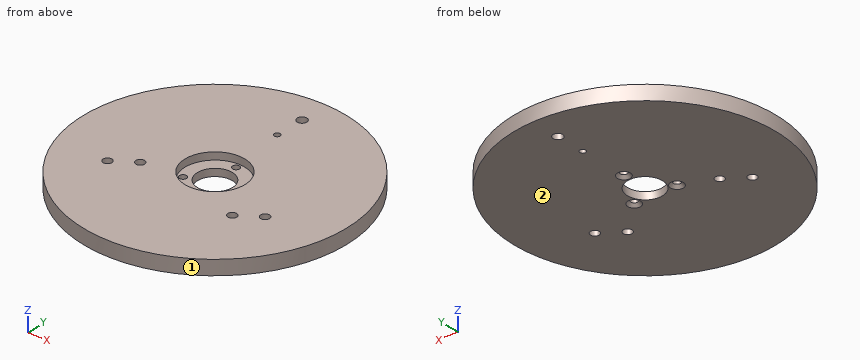
from build123d import *

# Parameters (mm, degrees)
SKETCH1_R                                       = 45
BOSS_EXTRUDE1_DEPTH                             = 5
F_20_5_20_5_DIAMETER_HOLE1_D                    = 20.5
F_20_5_20_5_DIAMETER_HOLE1_DEPTH                = 2.5
F_12_0_12_DIAMETER_HOLE1_D                      = 12
CSK_FOR_M2_FLAT_HEAD_MACHINE_SCREW1_D           = 2.4
CSK_FOR_M2_FLAT_HEAD_MACHINE_SCREW1_DEPTH       = 22.75
CSK_FOR_M2_FLAT_HEAD_MACHINE_SCREW1_CSINK_D     = 4.4
CSK_FOR_M2_FLAT_HEAD_MACHINE_SCREW1_CSINK_ANGLE = 90
CSK_FOR_M2_FLAT_HEAD_MACHINE_SCREW1_TIP         = 0.721032743
M4X0_7_TAPPED_HOLE1_D                           = 3.3
SKETCH15_R                                      = 1.5
M3_TAPPED_HOLE_DEPTH                            = 124.895116934
SKETCH16_R                                      = 1
F_2MM_PIN_DEPTH                                 = 124.895116934


with BuildPart() as part:
    # Sketch1 → Boss-Extrude1 (new body)
    with BuildSketch(Plane.XY.offset(39.5)):
        with Locations((-40, 45)):
            Circle(SKETCH1_R)
    extrude(amount=-BOSS_EXTRUDE1_DEPTH)

    # Ø20.5 (20.5) Diameter Hole1
    with Locations(Plane.XY.offset(39.5)):
        with Locations((-40, 45)):
            Hole(F_20_5_20_5_DIAMETER_HOLE1_D / 2, depth=F_20_5_20_5_DIAMETER_HOLE1_DEPTH)

    # Ø12.0 (12) Diameter Hole1 (through all)
    with Locations(Plane.XY.offset(39.5)):
        with Locations((-40, 45)):
            Hole(F_12_0_12_DIAMETER_HOLE1_D / 2)

    # CSK for M2 Flat Head Machine Screw1
    with Locations(Plane(origin=(0, 0, 34.5), x_dir=(1, 0, 0), z_dir=(0, 0, -1))):
        with Locations((-40, -53.5), (-32.638784068, -40.75), (-47.361215932, -40.75)):
            CounterSinkHole(CSK_FOR_M2_FLAT_HEAD_MACHINE_SCREW1_D / 2, CSK_FOR_M2_FLAT_HEAD_MACHINE_SCREW1_CSINK_D / 2, depth=CSK_FOR_M2_FLAT_HEAD_MACHINE_SCREW1_DEPTH, counter_sink_angle=CSK_FOR_M2_FLAT_HEAD_MACHINE_SCREW1_CSINK_ANGLE)
            with Locations((0, 0, -(CSK_FOR_M2_FLAT_HEAD_MACHINE_SCREW1_DEPTH + CSK_FOR_M2_FLAT_HEAD_MACHINE_SCREW1_TIP / 2))):  # 118° drill point
                Cone(0, CSK_FOR_M2_FLAT_HEAD_MACHINE_SCREW1_D / 2, CSK_FOR_M2_FLAT_HEAD_MACHINE_SCREW1_TIP, mode=Mode.SUBTRACT)

    # M4x0.7 Tapped Hole1 (through all)
    with Locations(Plane.XY.offset(39.5)):
        with Locations((-40, 80)):
            Hole(M4X0_7_TAPPED_HOLE1_D / 2)

    # Sketch15 → M3 Tapped Hole (cut, through all)
    with BuildSketch(Plane.XY.offset(39.5)):
        with Locations((-58, 36)):
            Circle(SKETCH15_R)
        with Locations((-65, 31)):
            Circle(SKETCH15_R)
        with Locations((-15, 36)):
            Circle(SKETCH15_R)
        with Locations((-22, 31)):
            Circle(SKETCH15_R)
    extrude(amount=-M3_TAPPED_HOLE_DEPTH, mode=Mode.SUBTRACT)

    # Sketch16 → 2mm Pin (cut, through all)
    with BuildSketch(Plane.XY.offset(39.5)):
        with Locations((-40, 70)):
            Circle(SKETCH16_R)
    extrude(amount=-F_2MM_PIN_DEPTH, mode=Mode.SUBTRACT)


solid = part.part
Geometry: final body of the model. Coordinates: model frame, mm. Face numbers are marked on the shaded views. Give positions to 0.01 mm unless a question says otherwise; leave off trailing zeros. Loops run counter-clockwise (first coordinate to the right, second up) from the corner with the lowest first, then second, coordinate; pieces in that order, holes last. Notation, with made-up numbers: (74, 65) - (109, 65) arc R14 cw to (109, 78) - close; hole circle Ø6 at (76.5, 78). An arc over 180 degrees is marked (long way). One line per question, with ' | ' between items. Start each with the question number.
(1) Pull-direction query (Y, two-part tool) for the marked faces 1 and 2; classes: released by +Y, released by -Y, zero draft, split by the parting line, or undercut.
(2) Section query C-C on x = -58. Return loops of the section in (y, z).
(3) Contact query for flat-ended pins moving along their axis: pin 1 (2 mm diameter, centred on x = -47.36, y = 40.75, fed in from -Z); pin 2 (1 mm diameter, centred on x = -75, z = 38, fed in from -Y); pin 3 (5 mm diameter, centred on x = -58, y = 36, fed in from +Z). Output: stop coordinate, or through.
(4) Section query B-B on y = 45. Return loops of the section in (x, z).
(5) Section query D-D on y = 36. Return loops of the section in (x, z), then the cut area to 3 significant figures.
(6) Section query A-A on z = 38.55. Return loops of the section in (x, y).
(7) Ray query, line 1 (X direction, y = 40.75, z = 36.3); line 2 (Y direction, x = -40, z = 37.05); line 3 (Y direction, x = -58, z = 37.3). Return the intervals inside material, ascending. Write a range as from..to.
The answers:
1) face 1: split by the parting line | face 2: zero draft
2) outline: (3.76, 34.5) - (34.5, 34.5) - (34.5, 39.5) - (3.76, 39.5) - close; (37.5, 34.5) - (86.24, 34.5) - (86.24, 39.5) - (37.5, 39.5) - close
3) pin 1: through | pin 2: y = 16.11 | pin 3: z = 39.5
4) outline: (-85, 34.5) - (-46, 34.5) - (-46, 37) - (-50.25, 37) - (-50.25, 39.5) - (-85, 39.5) - close; (-34, 34.5) - (5, 34.5) - (5, 39.5) - (-29.75, 39.5) - (-29.75, 37) - (-34, 37) - close
5) outline: (-84.09, 34.5) - (-59.5, 34.5) - (-59.5, 39.5) - (-84.09, 39.5) - close; (-56.5, 34.5) - (-16.5, 34.5) - (-16.5, 39.5) - (-35.09, 39.5) - (-35.09, 37) - (-44.91, 37) - (-44.91, 39.5) - (-56.5, 39.5) - close; (-13.5, 34.5) - (4.09, 34.5) - (4.09, 39.5) - (-13.5, 39.5) - close | area: 386 mm2
6) outline: circle Ø90 at (-40, 45); hole circle Ø3 at (-65, 31); hole circle Ø3 at (-58, 36); hole circle Ø20.5 at (-40, 45); hole circle Ø3.3 at (-40, 80); hole circle Ø2 at (-40, 70); hole circle Ø3 at (-22, 31); hole circle Ø3 at (-15, 36)
7) line 1: -84.8..-48.56, -46.16..-44.24, -35.76..-33.84, -31.44..4.8 | line 2: 0..34.75, 55.25..69, 71..78.35, 81.65..90 | line 3: 3.76..34.5, 37.5..86.24
